from build123d import *

# Parameters (mm, degrees)
BOSS_EXTRUDE1_DEPTH = 5
SKETCH3_W           = 56.45
SKETCH3_H           = 59.5
SKETCH3_R           = 1.85
BOSS_EXTRUDE3_DEPTH = 5
FILLET2_RADIUS      = 29.75
FILLET2_LENGTH      = 5


with BuildPart() as part:
    # Sketch1 → Boss-Extrude1 (new body)
    with BuildSketch(Plane.XY):
        Polygon((-31, 29.75), (-21, 29.75), (21, 29.75), (31, 29.75), (31, -29.75), (21, -29.75), (-21, -29.75), (-31, -29.75), align=None)
        with BuildLine():
            Line((-22.100164481, 6.625), (-21, 6.625))
            Line((-21, 6.625), (-21, 10.75))
            Line((-21, 10.75), (21.035787675, 10.75))
            Line((21.035787675, 10.75), (21, 6.625))
            Line((21, 6.625), (22.100164481, 6.625))
            ThreePointArc((22.100164481, 6.625), (26.5, 5), (22.100164481, 3.375))
            Line((22.100164481, 3.375), (21, 3.375))
            Line((21, 3.375), (21, -3.375))
            Line((21, -3.375), (22.100164481, -3.375))
            ThreePointArc((22.100164481, -3.375), (26.5, -5), (22.100164481, -6.625))
            Line((22.100164481, -6.625), (21, -6.625))
            Line((21, -6.625), (21, -10.75))
            Line((21, -10.75), (-21, -10.75))
            Line((-21, -10.75), (-21, -6.625))
            Line((-21, -6.625), (-22.100164481, -6.625))
            ThreePointArc((-22.100164481, -6.625), (-26.5, -5), (-22.100164481, -3.375))
            Line((-22.100164481, -3.375), (-21, -3.375))
            Line((-21, -3.375), (-21, 3.375))
            Line((-21, 3.375), (-22.100164481, 3.375))
            ThreePointArc((-22.100164481, 3.375), (-26.5, 5), (-22.100164481, 6.625))
        make_face(mode=Mode.SUBTRACT)
    extrude(amount=BOSS_EXTRUDE1_DEPTH)

    # Sketch3 → Boss-Extrude3 (add)
    with BuildSketch(Plane.ZY.offset(31)):
        with Locations((-23.225, 0)):
            Rectangle(SKETCH3_W, SKETCH3_H)
        with Locations(Location((-41.45, 19.75, 0), (0, 0, 270))):
            Circle(SKETCH3_R, mode=Mode.SUBTRACT)
        with Locations(Location((-41.45, -19.75, 0), (0, 0, 90))):
            Circle(SKETCH3_R, mode=Mode.SUBTRACT)
        with Locations(Location((-10.25, -19.75, 0), (0, 0, 270))):
            Circle(SKETCH3_R, mode=Mode.SUBTRACT)
        with Locations(Location((-10.25, 19.75, 0), (0, 0, 90))):
            Circle(SKETCH3_R, mode=Mode.SUBTRACT)
    extrude(amount=BOSS_EXTRUDE3_DEPTH)

    # Fillet2: full round fillet: the end face becomes a half cylinder, R = half its width
    fillet2_face = Plane((31, 0, 2.5), x_dir=(0, 0, 1), z_dir=(1, 0, 0))  # on the end face: x along it, z out of the body
    fillet2_slab = fillet2_face.offset(-FILLET2_RADIUS / 2) * Box(FILLET2_LENGTH, 2 * FILLET2_RADIUS, FILLET2_RADIUS, mode=Mode.PRIVATE)  # the body's end, R deep
    fillet2_round = Plane((1.25, 0, 2.5), x_dir=(1, 0, 0), z_dir=(0, 0, 1)) * Cylinder(FILLET2_RADIUS, FILLET2_LENGTH, mode=Mode.PRIVATE)  # its axis R under the face
    add(fillet2_slab - fillet2_round, mode=Mode.SUBTRACT)


solid = part.part
The listing builds one solid part. Answer for the finished solid, in the listing's coordinates (mm). A direction names the side the tool comes from. Coordinates: 2 decimals unless noted, no trailing zeros. Loops run counter-clockwise (first coordinate to the right, second up) from the corner with the lowest first, then second, coordinate; pieces in that order, holes last. Notation, with made-up numbers: M 14.25,-35 L 58.25,-35 A9 ccw 58.25,-26 Z; hole C 19.25,-39.75 d5. An arc over 180 degrees is marked long. Answer in a Markdown table with one row per item.
1) Find section C-C (x = 8). Determine the outline of the cut face in (y, z).
Answers below:
| item | result |
|---|---|
| outline | M -28.97,0 L -10.75,0 L -10.75,5 L -28.97,5 Z; M 10.75,0 L 28.97,0 L 28.97,5 L 10.75,5 Z |
2) Find section A-A (z = -10.25). Determine the outline of the cut face in (x, y).
Answers below:
| item | result |
|---|---|
| outline | M -36,-29.75 L -31,-29.75 L -31,-21.6 L -36,-21.6 Z; M -36,-17.9 L -31,-17.9 L -31,17.9 L -36,17.9 Z; M -36,21.6 L -31,21.6 L -31,29.75 L -36,29.75 Z |
3) Find section B-B (y = 19.75). Determine the outline of the cut face in (x, z).
Answers below:
| item | result |
|---|---|
| outline | M -36,-51.45 L -31,-51.45 L -31,-43.3 L -36,-43.3 Z; M -36,-39.6 L -31,-39.6 L -31,-12.1 L -36,-12.1 Z; M -36,-8.4 L -31,-8.4 L -31,0 L 23.5,0 L 23.5,5 L -36,5 Z |
4) Which of the six approach directions +Z, -Z, +X, -X, +Y, -Y give full straight-line access (tool end or side, diameter ignored) to faces 4 (the flat face through (-31, 0, -26)), 5 (the flat face through (-21, 0, 2)), 6 (the flat face through (-36, 0, -24))?
Answers below:
| item | result |
|---|---|
| face 4 | -Z, +X, +Y, -Y |
| face 5 | +Z, -Z |
| face 6 | +Z, -Z, -X, +Y, -Y |
5) Given pin 1 (0.6 mm diameter, centred on x = 21.5, z = 2, fed in from +Y); pin 2 (5.5 mm diameter, centred on x = -24, y = -5, fed in from -Z); pin 3 (12 mm diameter, centred on x = 20.5, z = -9, fed in from +Y); pin 4 (2 mm diameter, centred on y = 16.5, z = -6.5, fed in from +X), each flat-ended and moving along its own axis, determine where each tip first touches the part or whether it passes through.
Answers below:
| item | result |
|---|---|
| pin 1 | y = 22.07 |
| pin 2 | z = 0 |
| pin 3 | through |
| pin 4 | x = -31 |
6) Determine the mould class of faces 1 (the flat face through (0, -10.75, 2)), 2 (the flat face through (-9, 13, 5)), 3 (the flat face through (-21, -9, 2)) for opening direction Y: released by +Y, released by -Y, zero draft, split by the parting line, or undercut.
Answers below:
| item | result |
|---|---|
| face 1 | undercut |
| face 2 | zero draft |
| face 3 | undercut |
7) Find the intervals of material crossed by probe 1 along Z at (x, y) = (-34.9, 19.75); probe 2 along Z at (x, y) = (-23, -18); probe 3 along X at (y, z) = (26.5, -36), in increasing order.
Answers below:
| item | result |
|---|---|
| probe 1 | -51.45 to -43.3, -39.6 to -12.1, -8.4 to 5 |
| probe 2 | 0 to 5 |
| probe 3 | -36 to -31 |
8) Find section D-D (x = 24). Determine the outline of the cut face in (y, z), then the cut area to 3 significant figures.
Answers below:
| item | result |
|---|---|
| outline | M -19.17,0 L -7.5,0 L -7.5,5 L -19.17,5 Z; M -2.5,0 L 2.5,0 L 2.5,5 L -2.5,5 Z; M 7.5,0 L 19.17,0 L 19.17,5 L 7.5,5 Z |
| area | 142 mm^2 |
